Could you check a few things on this drawing? It's one solid part, dimensions in mm from its lowest x, y, z. A direction names the side the tool comes from. Round coordinates to 2 decimals unless told otherwise and drop trailing zeros. Write each loop counter-clockwise with the first axis right and the second up, starting at its lowest first coordinate (ties: lowest second). Pieces come first, ordered by that corner, then holes. Notation, with made-up numbers: (1.25, 18.25) -> (39.25, 18.25) arc R8 ccw to (39.25, 24.25) -> close; hole circle Ø2 at (-2.5, -23). An arc over 180 degrees is marked (long way). Answer as CSV lines item,"result".
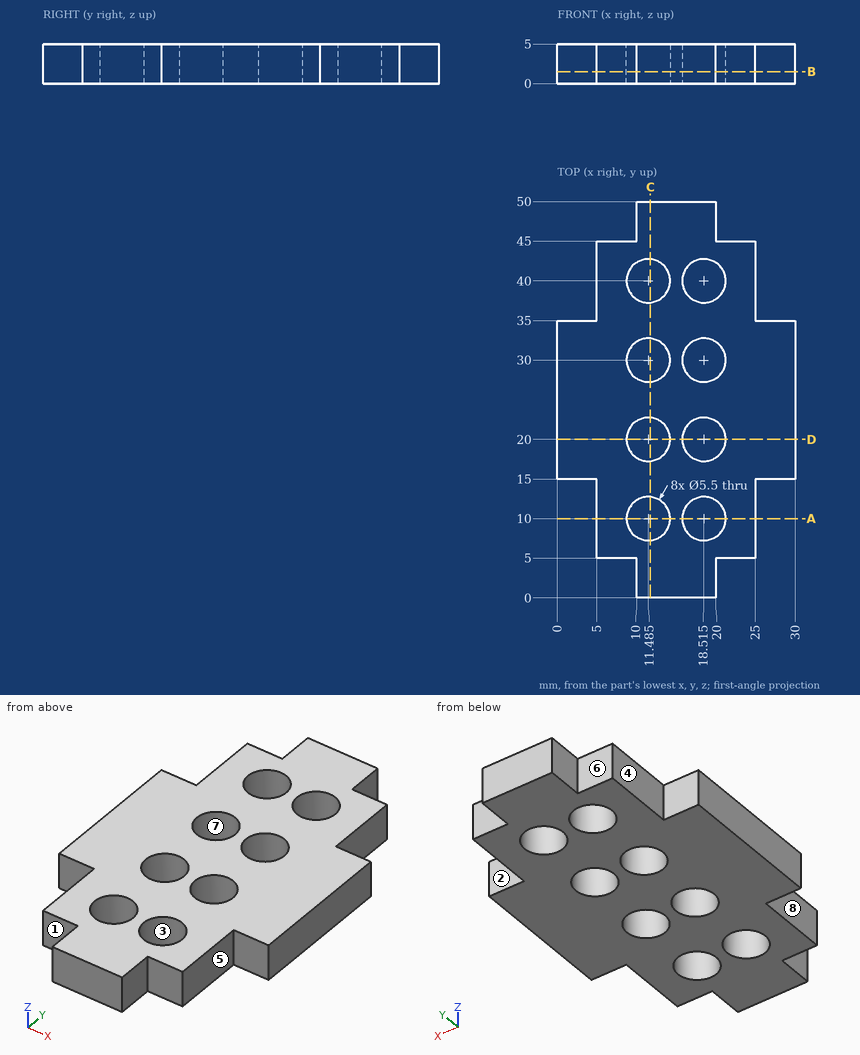
1. Suppose I cut it at D-D on y = 20. Please give me the cut outline in (x, z) (3 decimals), and give its area (3 significant figures).
Numbers:
outline,"(0, 0) -> (8.735, 0) -> (8.735, 5) -> (0, 5) -> close; (14.235, 0) -> (15.765, 0) -> (15.765, 5) -> (14.235, 5) -> close; (21.265, 0) -> (30, 0) -> (30, 5) -> (21.265, 5) -> close"
area,"95.0 mm^2"
2. For pin 1 Ø7 at (x, y) = (18.52, 10) entering from -Z; pin 2 Ø2.5 at (y, z) = (46.5, 3) entering from -X; pin 3 Ø2.5 at (y, z) = (9, 2.5) entering from +X; pin 4 Ø3.5 at (x, y) = (11.48, 10) entering from -Z, each with a flat end and sliding along its axis, tell me the tip position at first contact or that it passes through.
Numbers:
pin 1,"stops at z = 0"
pin 2,"stops at x = 10"
pin 3,"stops at x = 25"
pin 4,"passes through"
3. Suppose I cut it at B-B on z = 1.5. Count the separate pieces of the cut face and the enclosed holes in it, and give its area (3 significant figures).
Numbers:
separate pieces,"1"
enclosed holes,"8"
area,"910 mm^2"
4. Suppose I cut it at A-A on y = 10. Please give me the cut outline in (x, z) (3 decimals), and give its area (3 significant figures).
Numbers:
outline,"(5, 0) -> (8.735, 0) -> (8.735, 5) -> (5, 5) -> close; (14.235, 0) -> (15.765, 0) -> (15.765, 5) -> (14.235, 5) -> close; (21.265, 0) -> (25, 0) -> (25, 5) -> (21.265, 5) -> close"
area,"45.0 mm^2"
5. If we mould it in two halves opening along Y, with no side actions, what happens to the marked faces 6, 7 and 8? For each: released by +Y, released by -Y, zero draft, split by the parting line, or undercut.
Numbers:
face 6,"released by +Y"
face 7,"undercut"
face 8,"zero draft"
6. If I drill on line 1 (X direction, y = 22, z = 0.85); line 2 (Y direction, x = 11, z = 2.8); line 3 (X direction, y = 12, z = 2.8), over which ranges is the centre line in solid material (lowest first)?
Numbers:
line 1,"x = 0 to 9.6, 13.37 to 16.63, 20.4 to 30"
line 2,"y = 0 to 7.29, 12.71 to 17.29, 22.71 to 27.29, 32.71 to 37.29, 42.71 to 50"
line 3,"x = 5 to 9.6, 13.37 to 16.63, 20.4 to 25"
7. Suppose I cut it at C-C on x = 11.75. Please give me the cut outline in (y, z).
Numbers:
outline,"(0, 0) -> (7.26, 0) -> (7.26, 5) -> (0, 5) -> close; (12.74, 0) -> (17.26, 0) -> (17.26, 5) -> (12.74, 5) -> close; (22.74, 0) -> (27.26, 0) -> (27.26, 5) -> (22.74, 5) -> close; (32.74, 0) -> (37.26, 0) -> (37.26, 5) -> (32.74, 5) -> close; (42.74, 0) -> (50, 0) -> (50, 5) -> (42.74, 5) -> close"
8. On a 3-axis mill with a long thin cutter (end or side, diameter ignored), from which of +Z, -Z, +X, -X, +Y, -Y can I reach the whole of each face in a straight line? I mean the marked faces 1, 2, 3, 4 and 5. Say none if no direction works.
Numbers:
face 1,"+Z, -Z, -X, -Y"
face 2,"+Z, -Z, +X, +Y"
face 3,"+Z, -Z"
face 4,"+Z, -Z, -X, +Y"
face 5,"+Z, -Z, +X, -Y"
